Read the model definition and answer for the solid it produces. Units are mm, in the model's axes. Face numbers are marked on the shaded views. Round coordinates to 2 decimals unless told otherwise and drop trailing zeros. Write each loop counter-clockwise with the first axis right and the second up, starting at its lowest first coordinate (ties: lowest second). Pieces come first, ordered by that corner, then holes.
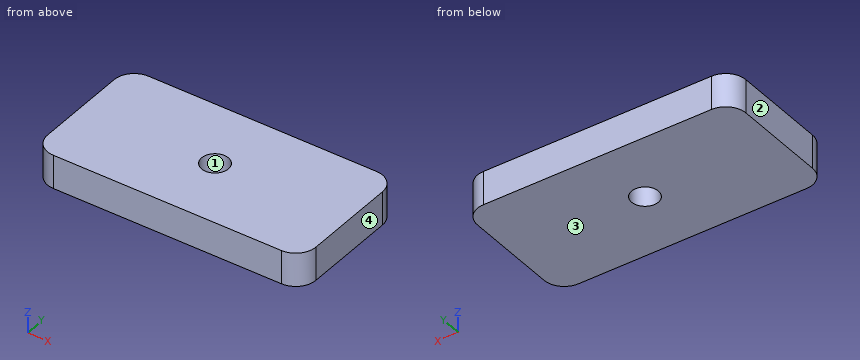
from build123d import *

# Parameters (mm, degrees)
BOSS_EXTRUDE1_DEPTH = 5
CUT_EXTRUDE1_REACH  = 24.913
SKETCH2_R           = 2


with BuildPart() as part:
    # Sketch1 → Boss-Extrude1 (new body)
    with BuildSketch(Plane.XY):
        with BuildLine():
            Line((17, 10), (-17, 10))
            ThreePointArc((-17, 10), (-19.121320344, 9.121320344), (-20, 7))
            Line((-20, 7), (-20, -7))
            ThreePointArc((-20, -7), (-19.121320344, -9.121320344), (-17, -10))
            Line((-17, -10), (17, -10))
            ThreePointArc((17, -10), (19.121320344, -9.121320344), (20, -7))
            Line((20, -7), (20, 7))
            ThreePointArc((20, 7), (19.121320344, 9.121320344), (17, 10))
        make_face()
    extrude(amount=BOSS_EXTRUDE1_DEPTH)

    # Sketch2 → Cut-Extrude1 (cut, up to next)
    with BuildSketch(Plane(origin=(0, 0, 0), x_dir=(-1, 0, 0), z_dir=(0, 0, -1)), mode=Mode.PRIVATE) as cut_extrude1_sk1:
        Circle(SKETCH2_R)
    cut_extrude1_tool1 = extrude(cut_extrude1_sk1.sketch, amount=-CUT_EXTRUDE1_REACH, mode=Mode.PRIVATE) & part.part
    add(cut_extrude1_tool1.solids().sort_by_distance((0, 0, 0))[0], mode=Mode.SUBTRACT)


solid = part.part
Q1. Straight lines are drawn through the part: probe 1 along Y at (x, z) = (0, 3.05); probe 2 along X at (y, z) = (-0.75, 3.85); probe 3 along X at (y, z) = (9, 2). For each, find the intervals that lie inside material, in ascending order.
Verdict:
probe 1: y = -10 to -2, 2 to 10
probe 2: x = -20 to -1.85, 1.85 to 20
probe 3: x = -19.24 to 19.24
Q2. Section C-C (z = 2.1) is taken. Determine the outline of the cut face in (x, y), then the cut area to 3 significant figures.
Verdict:
outline: (-20, -7) arc R3 ccw to (-17, -10) - (17, -10) arc R3 ccw to (20, -7) - (20, 7) arc R3 ccw to (17, 10) - (-17, 10) arc R3 ccw to (-20, 7) - close; hole circle Ø4 at (0, 0)
area: 780 mm2
Q3. Determine the mould class of the marked faces 1, 2, 3 and 4 for opening direction X: pulls with the +X half, pulls with the -X half, needs draft (parallel to the pull), parting line crosses it, or undercut.
Verdict:
face 1: undercut
face 2: pulls with the -X half
face 3: needs draft
face 4: pulls with the +X half
Q4. Section B-B (x = 0) is taken. Determine the outline of the cut face in (y, z), then the cut area to 3 significant figures.
Verdict:
outline: (-10, 0) - (-2, 0) - (-2, 5) - (-10, 5) - close; (2, 0) - (10, 0) - (10, 5) - (2, 5) - close
area: 80.0 mm2
Q5. Section A-A (y = 0) is taken. Determine the outline of the cut face in (x, z).
Verdict:
outline: (-20, 0) - (-2, 0) - (-2, 5) - (-20, 5) - close; (2, 0) - (20, 0) - (20, 5) - (2, 5) - close
